Drawing for the job (mm, zero at the part's lowest x, y, z). A direction names the side the tool comes from. Give positions to 0.01 mm unless a question says otherwise; leave off trailing zeros. Order: outer loops, then holes, each group sorted by start corner. A loop starts at its lowest first (then second) coordinate and runs counter-clockwise, first axis right, second up. Notation, with made-up numbers: (30.5, 38.5) - (85.5, 38.5) arc R8 ccw to (85.5, 45.5) - close; hole circle Ø5 at (3, 7.25). An arc over 180 degrees is marked (long way). Use CSV: the item, a comma, the result in double quotes. Start each with the question number.
(1) Band-saw the part on A-A, the plane y = 45. Count the separate pieces of the cut face and the enclosed holes in it, then the cut area to 3 significant figures.
(2) Band-saw the part on B-B, the plane y = 39. Give the cut face in (x, z) (1 decimal), then the cut area to 3 significant figures.
(3) Band-saw the part on D-D, the plane x = 47. Give the cut face in (y, z).
(4) Drop flat-ended pins along their axis: pin 1 Ø1.5 at (x, y) = (8.5, 44) entering from +Z; pin 2 Ø11.5 at (x, y) = (29.5, 35.5) entering from +Z; pin 3 Ø2 at (y, z) = (16, 28.5) entering from +X; pin 4 Ø3.5 at (x, y) = (47.5, 29.5) entering from -Z. Give the stop position or say it passes through.
(5) Probe L1, parallel to Y at x = 47, z = 18; L2, parallel to X at y = 19.5, z = 20; L3, parallel to Z at x = 27, y = 17. List the from-to ranges inside material, lowest first.
(6) Tool access for the marked faces 1, 2, 3 and 4: list every direction of +Z, -Z, +X, -X, +Y, -Y with a clear straight run to the whole face (end or side of a thin tool).
(7) Band-saw the part on C-C, the plane z = 26.5. Give the cut face in (x, y), then the cut area to 4 significant figures.
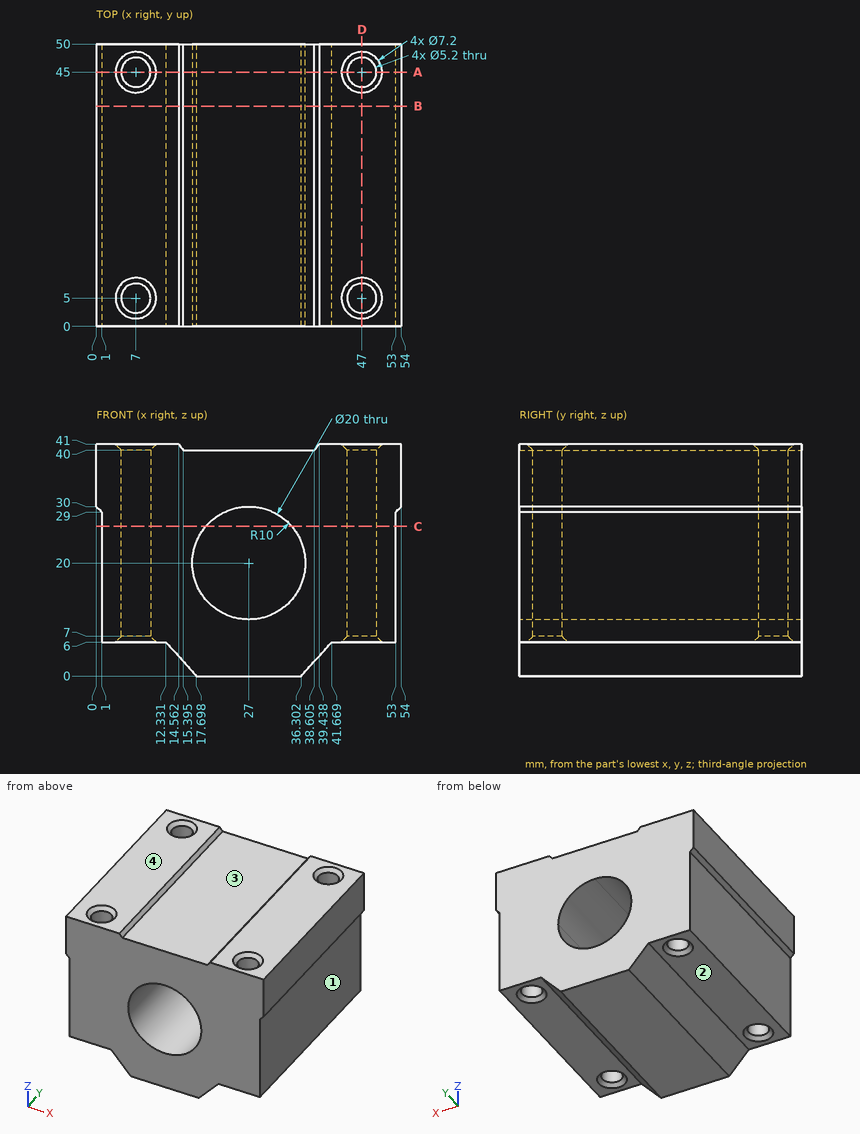
Answer block:
1,separate pieces,"3"
1,enclosed holes,"1"
1,area,"1,280 mm2"
2,outline,"(0, 30) - (1, 29) - (1, 6) - (12.3, 6) - (17.7, 0) - (36.3, 0) - (41.7, 6) - (53, 6) - (53, 29) - (54, 30) - (54, 41) - (39.4, 41) - (38.6, 40) - (15.4, 40) - (14.6, 41) - (0, 41) - close; hole circle Ø20 at (27, 20)"
2,area,"1,650 mm2"
3,outline,"(0, 6) - (1.4, 6) - (2.4, 7) - (2.4, 40) - (1.4, 41) - (0, 41) - close; (7.6, 7) - (8.6, 6) - (41.4, 6) - (42.4, 7) - (42.4, 40) - (41.4, 41) - (8.6, 41) - (7.6, 40) - close; (47.6, 7) - (48.6, 6) - (50, 6) - (50, 41) - (48.6, 41) - (47.6, 40) - close"
4,pin 1,"passes through"
4,pin 2,"stops at z = 40"
4,pin 3,"stops at x = 53.5"
4,pin 4,"stops at z = 6"
5,L1,"y = 0 to 2.4, 7.6 to 42.4, 47.6 to 50"
5,L2,"x = 1 to 17, 37 to 53"
5,L3,"z = 0 to 10, 30 to 40"
6,face 1,"-Z, +X, +Y, -Y"
6,face 2,"-Z, -X, +Y, -Y"
6,face 3,"+Z, +Y, -Y"
6,face 4,"+Z, +X, -X, +Y, -Y"
7,outline,"(1, 0) - (19.4, 0) - (19.4, 50) - (1, 50) - close; (34.6, 0) - (53, 0) - (53, 50) - (34.6, 50) - close; hole circle Ø5.2 at (7, 5); hole circle Ø5.2 at (7, 45); hole circle Ø5.2 at (47, 5); hole circle Ø5.2 at (47, 45)"
7,area,"1,755 mm2"
